Design review of the part built by this model. Coordinates are the model's own, in mm. A direction names the side the tool comes from. Coordinates: 2 decimals unless noted, no trailing zeros. Write each loop counter-clockwise with the first axis right and the second up, starting at its lowest first coordinate (ties: lowest second). Pieces come first, ordered by that corner, then holes. Notation, with made-up numbers: (35.5, 21.5) - (94.5, 21.5) arc R14 ccw to (94.5, 25.5) - close; hole circle Ø2 at (85, 63.5). An arc over 180 degrees is marked (long way). One line per item, written item: value.
Autodesk Inventor part; units mm, degrees
ref_plane "YZ Plane" through (0, 0, 0) normal (1, 0, 0) x (0, 1, 0)
ref_plane "XZ Plane" through (0, 0, 0) normal (0, 1, 0) x (-1, 0, 0)
ref_plane "XY Plane" through (0, 0, 0) normal (0, 0, 1) x (1, 0, 0)
sketch "Sketch1" plane through (0, 0, 0) normal (0, 0, 1) x (1, 0, 0)
  line L0 (25, 15) -> (-25, 15)
  line L1 (-25, 15) -> (-25, -15)
  line L2 (-25, -15) -> (25, -15)
  line L3 (25, -15) -> (25, 15)
  line L4 (25, 15) -> (-25, -15) construction
  line L5 (-25, 15) -> (25, -15) construction
  point P0 (0, 0)
  dimension "d0" = 50
  dimension "d1" = 30
extrude "Extrusion1" add sketch "Sketch1" along normal blind 4
fillet "Fillet1" radius 1 1 edges at (25, 15, 2)
fillet "Fillet2" radius 1 3 edges at (-25, 15, 2) (25, -15, 2) (-25, -15, 2)
sketch "Sketch4" plane through (0, 0, 4) normal (0, 0, 1) x (1, 0, 0)
  circle A0 centre (0, 0) radius 1.5
  dimension "d19" = 3
hole "Hole2" at (0, 0, 4) direction (0, 0, -1) diameter 3 end through all both
sketch "Sketch6" plane through (0, 0, 4) normal (0, 0, 1) x (1, 0, 0)
  circle A0 centre (-20, 11) radius 2.5
  circle A1 centre (20, 11) radius 2.5
  circle A2 centre (-20, -11) radius 2.5
  circle A3 centre (20, -11) radius 2.5
  line L0 (25, -14) -> (25, 14)
  line L1 (-25, 14) -> (-25, -14)
  line L2 (24, 15) -> (-24, 15)
  line L3 (-24, -15) -> (24, -15)
  point P0 (0, 0)
  dimension "d27" = 5
  dimension "d28" = 5
  dimension "d29" = 5
  dimension "d30" = 5
  dimension "d38" = 5
  dimension "d39" = 5
  dimension "d40" = 5
  dimension "d41" = 5
  dimension "d42" = 4
  dimension "d43" = 4
  dimension "d44" = 4
  dimension "d45" = 4
sketch "Sketch18" plane through (0, 0, 0) normal (0, 0, -1) x (-1, 0, 0)
  point P0 (0, 0)
extrude "Extrusion10" add sketch "Sketch6" against normal blind 12
sketch "Sketch19" plane through (0, 0, 0) normal (0, 0, -1) x (-1, 0, 0)
  line L0 (24, -15) -> (-24, -15)
  line L1 (-9, -15) -> (9, -15)
  line L2 (9, -15) -> (9, -21)
  line L3 (9, -21) -> (-9, -21)
  line L4 (-9, -21) -> (-9, -15)
  point P0 (0, 0)
  dimension "d84" = 18
  dimension "d85" = 6
extrude "Extrusion11" add sketch "Sketch19" against normal blind 26
sketch "Sketch20" plane through (-9, -15, 4) normal (0, 1, 0) x (1, 0, 0)
  point P0 (9, 4)
sketch "Sketch21" plane through (-9, -15, 4) normal (0, 1, 0) x (1, 0, 0)
  line L0 (33, 0) -> (-15, 0)
  line L1 (3, 0) -> (15, 0)
  line L2 (15, 0) -> (15, -19)
  line L3 (15, -19) -> (3, -19)
  line L4 (3, -19) -> (3, 0)
  point P0 (9, 4)
  dimension "d88" = 12
  dimension "d89" = 19
extrude "Extrusion12" cut sketch "Sketch21" against normal blind 3
fillet "Fillet11" radius 3 3 edges at (-9, -15, 15) (9, -15, 15) (0, -15, 26)
properties part number "reward v06"
1. Insertion check: pin 1 Ø2.5 at (x, y) = (0, 0) entering from -Z; pin 2 Ø3.5 at (y, z) = (-17, 16) entering from +X; pin 3 Ø11 at (x, y) = (-6.5, -11) entering from -Z; pin 4 Ø13 at (x, z) = (-2.5, 17.5) entering from +Y. Each pin has a flat end and moves straight along its axis. Give the tip position at first contact, or say it passes through.
Answer block:
pin 1: passes through
pin 2: stops at x = 9
pin 3: stops at z = 0
pin 4: stops at y = -15
2. Wall thickness on line 1 along Y through (x, z) = (0, 1); line 2 along X through (y, z) = (0, 3.1); line 3 along Z through (x, y) = (-10, -13): over which ranges is each line inside the solid? List them lowest first.
Answer block:
line 1: y = -21 to -1.5, 1.5 to 15
line 2: x = -25 to -1.5, 1.5 to 25
line 3: z = 0 to 4
3. For faces 5 (the face through (-8.1, -15.86, 15.15)), 6 (the face through (16, -15, 2)), 7 (the face through (-6, -16, 14)), 8 (the face through (-22, 9.5, -3.9)), list the 3-axis set-ups (+Z, -Z, +X, -X, +Y, -Y) from which the entire face can be reached by the end or side of a thin tool; tool diameter is ignored.
Answer block:
face 5: +Z, -X, +Y
face 6: +Z, -Z, +X, -Y
face 7: +Y
face 8: -Z
4. Mouldability with a two-part tool opening along X and no side actions: class faces 1 (the face through (-9, -19, 13)), 2 (the face through (18, 9.5, -3.9)), 3 (the face through (9, -19, 13)), 4 (the face through (6, -16, 13)) as released by +X, released by -X, zero draft, split by the parting line, or undercut.
Answer block:
face 1: released by -X
face 2: undercut
face 3: released by +X
face 4: undercut
5. Consider section B-B, the plane y = 0. Write out the cut boundary in (x, z).
Answer block:
outline: (-25, 0) - (-1.5, 0) - (-1.5, 4) - (-25, 4) - close; (1.5, 0) - (25, 0) - (25, 4) - (1.5, 4) - close
6. Consider section C-C, the plane y = -11. Write out the cut boundary in (x, z).
Answer block:
outline: (-25, 0) - (-22.5, 0) - (-22.5, -8) - (-17.5, -8) - (-17.5, 0) - (17.5, 0) - (17.5, -8) - (22.5, -8) - (22.5, 0) - (25, 0) - (25, 4) - (-25, 4) - close
